Source: CAD feature listing. Evaluate the final solid. Frame: model axes, mm. A direction names the side the tool comes from. Round coordinates to 2 decimals unless told otherwise and drop trailing zeros. Write each loop counter-clockwise with the first axis right and the second up, starting at its lowest first coordinate (ties: lowest second). Pieces come first, ordered by that corner, then holes. Notation, with made-up numbers: (44.25, 34) - (102.25, 34) arc R6 cw to (102.25, 38) - close; hole circle Ø8 at (12.5, 38.5). An arc over 180 degrees is marked (long way). Write item = value, one per line. Start each with the question number.
```python
from build123d import *

# Parameters (mm, degrees)
SKETCH1_W           = 32
SKETCH1_H           = 13
BOSS_EXTRUDE1_DEPTH = 24
SKETCH2_W           = 12
SKETCH2_H           = 13
CUT_EXTRUDE1_DEPTH  = 43.05948169
SKETCH3_R           = 4.5
CUT_EXTRUDE2_DEPTH  = 43.05948169
SKETCH4_R           = 12
BOSS_EXTRUDE2_DEPTH = 10
SKETCH5_R           = 5
CUT_EXTRUDE3_DEPTH  = 47.14108798
SKETCH6_R           = 5
CUT_EXTRUDE4_DEPTH  = 47.14108798


with BuildPart() as part:
    # Sketch1 → Boss-Extrude1 (new body)
    with BuildSketch(Plane.XY):
        with Locations((-16, 6.5)):
            Rectangle(SKETCH1_W, SKETCH1_H)
    boss_extrude1 = extrude(amount=BOSS_EXTRUDE1_DEPTH)

    # Sketch2 → Cut-Extrude1 (cut, through all)
    with BuildSketch(Plane(origin=(0, 0, 0), x_dir=(-1, 0, 0), z_dir=(0, 0, -1))):
        with Locations((16, 6.5)):
            Rectangle(SKETCH2_W, SKETCH2_H)
    cut_extrude1 = extrude(amount=-CUT_EXTRUDE1_DEPTH, mode=Mode.SUBTRACT)


with BuildPart() as cut_extrude1_piece_1:
    # of the separate pieces the step leaves, piece 1, a body of its own (cut_extrude1_pieces)
    add(part.part.solids().sort_by_distance((0, 0, 0))[0])


with BuildPart() as cut_extrude1_piece_2:
    # of the separate pieces the step leaves, piece 2, a body of its own (cut_extrude1_pieces)
    add(part.part.solids().sort_by_distance((-32, 0, 0))[0])


with BuildPart() as cut_extrude2_tool:
    # Sketch3 → Cut-Extrude2 (new, through all)
    with BuildSketch(Plane(origin=(0, 0, 0), x_dir=(0, 0, -1), z_dir=(1, 0, 0))):
        with Locations((-12, 6.5)):
            Circle(SKETCH3_R)
    cut_extrude2 = extrude(amount=-CUT_EXTRUDE2_DEPTH)


with BuildPart() as cut_extrude1_piece_1_1:
    add(cut_extrude1_piece_1.part)

    # Cut-Extrude2: cut by cut_extrude2_tool
    add(cut_extrude2_tool.part, mode=Mode.SUBTRACT)



with BuildPart() as cut_extrude1_piece_2_1:
    add(cut_extrude1_piece_2.part)

    # Cut-Extrude2: cut by cut_extrude2_tool
    add(cut_extrude2_tool.part, mode=Mode.SUBTRACT)


with BuildPart() as cut_extrude1_piece_1_2:
    add(cut_extrude1_piece_1_1.part)

    add(cut_extrude1_piece_2_1.part)  # Boss-Extrude2 merges Cut-Extrude1 piece 2
    # Sketch4 → Boss-Extrude2 (add)
    with BuildSketch(Plane(origin=(0, 0, 0), x_dir=(-1, 0, 0), z_dir=(0, -1, 0))):
        with Locations(Location((16, -12, 0), (0, 0, 240))):
            Circle(SKETCH4_R)
    extrude(amount=BOSS_EXTRUDE2_DEPTH)

    # Mirror1: Boss-Extrude1, Cut-Extrude1, Cut-Extrude2 across plane
    add(boss_extrude1.mirror(Plane.ZX.offset(-5)))
    add(cut_extrude1.mirror(Plane.ZX.offset(-5)), mode=Mode.SUBTRACT)
    add(cut_extrude2.mirror(Plane.ZX.offset(-5)), mode=Mode.SUBTRACT)

    # Sketch5 → Cut-Extrude3 (cut, through all)
    with BuildSketch(Plane(origin=(0, 0, 0), x_dir=(0, 0, -1), z_dir=(1, 0, 0))):
        with Locations((-12, -16.5)):
            Circle(SKETCH5_R)
    extrude(amount=-CUT_EXTRUDE3_DEPTH, mode=Mode.SUBTRACT)

    # Sketch6 → Cut-Extrude4 (cut, through all)
    with BuildSketch(Plane.ZY.offset(32)):
        with Locations((12, 6.5)):
            Circle(SKETCH6_R)
    extrude(amount=-CUT_EXTRUDE4_DEPTH, mode=Mode.SUBTRACT)


solid = cut_extrude1_piece_1_2.part
```
(1) Section C-C (z = 12). Count the separate pieces of the cut face and the enclosed holes in it, plus the area to 3 significant figures.
(2) Reachability of faces 1 (the flat face through (-22, 2, 9)), 2 (the flat face through (-28.2, 0, 11.8)), 3 (the flat face through (-3, -10, 12)), 4 (the flat face through (-16, -10, 12)) from +Z, -Z, +X, -X, +Y, -Y: full face, straight path, thin tool, end or side. Return the list, or none.
(3) Ray query, L1, parallel to Y at x = -6.25, z = 12; L2, parallel to Y at x = -2.75, z = 12; L3, parallel to Y at x = -29, z = 2.5. Return the intervals inside material, ascending. Write a range as from..to.
(4) Pull-direction query (Y, two-part tool) for faces 5 (the flat face through (-27, 7, 24)), 6 (the flat face through (-5, -23, 12)), 7 (the flat face through (-3, 0, 12)); classes: +Y half, -Y half, draft (parallel to the pull), parting line (faces both ways), or undercut.
(5) Section B-B (y = 6.5). Return the cut outline in (x, z).
(6) Section A-A (x = -2.5). Return the cut outline in (y, z).
(7) Section D-D (x = -27.5). Return the cut outline in (y, z).
(8) Contact query for flat-ended pins moving along their axis: P1, Ø6, axis at y = -16.5, z = 12, coming from the +X side; P2, Ø4, axis at x = -19, y = -0.5, coming from the +Z side; P3, Ø4, axis at y = -3.5, z = 7, coming from the +X side; P4, Ø6, axis at x = -18.5, z = 7.5, coming from the +Y side. Output: stop coordinate, or through.
Solution:
q1.separate_pieces = 5
q1.enclosed_holes = 0
q1.area = 360 mm^2
q2.face_1 = +Z, -Z, +Y
q2.face_2 = -X
q2.face_3 = +X
q2.face_4 = +Z, -Z, -Y
q3.L1 = -23..-21.5, -11.5..1.5, 11.5..13
q3.L2 = -23..-21.5, -11.5..-10, 0..1.5, 11.5..13
q3.L3 = -23..-10, 0..13
q4.face_5 = draft
q4.face_6 = -Y half
q4.face_7 = undercut
q5.outline = (-32, 0) - (-22, 0) - (-22, 7) - (-32, 7) - close; (-32, 17) - (-22, 17) - (-22, 24) - (-32, 24) - close; (-10, 0) - (0, 0) - (0, 7) - (-10, 7) - close; (-10, 17) - (0, 17) - (0, 24) - (-10, 24) - close
q6.outline = (-23, 0) - (-10, 0) - (-10, 24) - (-23, 24) - close; (0, 0) - (13, 0) - (13, 24) - (0, 24) - close; hole circle Ø10 at (-16.5, 12); hole circle Ø10 at (6.5, 12)
q7.outline = (-23, 0) - (-10, 0) - (-10, 8.57) - (0, 8.57) - (0, 0) - (13, 0) - (13, 24) - (0, 24) - (0, 15.43) - (-10, 15.43) - (-10, 24) - (-23, 24) - close; hole circle Ø10 at (-16.5, 12); hole circle Ø10 at (6.5, 12)
q8.P1 = through
q8.P2 = 23.96
q8.P3 = -4.38
q8.P4 = 0
